```python
from build123d import *

# Parameters (mm, degrees)
SKETCH1_W            = 110
SKETCH1_H            = 60
BOSS_EXTRUDE1_DEPTH  = 10
SKETCH2_W            = 93.6
SKETCH2_H            = 43.6
BOSS_EXTRUDE3_DEPTH  = 7
SKETCH3_W            = 22.1
SKETCH3_H            = 23.4
CUT_EXTRUDE1_DEPTH   = 7
FILLET1_R            = 12
FILLET1_OF_MIRROR1_R = 12
CUT_EXTRUDE3_START   = -10
CUT_EXTRUDE3_DEPTH   = 10


# Read off the part's stored shape, not the designer's step: Cut-Extrude3
with BuildPart() as part:
    # Sketch1 → Boss-Extrude1 (new body)
    with BuildSketch(Plane.XY):
        with Locations((55, 30)):
            Rectangle(SKETCH1_W, SKETCH1_H)
    extrude(amount=BOSS_EXTRUDE1_DEPTH)

    # Sketch2 → Boss-Extrude3 (add)
    with BuildSketch(Plane.XY.offset(10)):
        with Locations((55, 30)):
            Rectangle(SKETCH2_W, SKETCH2_H)
    extrude(amount=BOSS_EXTRUDE3_DEPTH)

    # Sketch3 → Cut-Extrude1 (cut)
    with BuildSketch(Plane.XY.offset(17)):
        with Locations((37.45, 19.9)):
            Rectangle(SKETCH3_W, SKETCH3_H)
    cut_extrude1 = extrude(amount=-CUT_EXTRUDE1_DEPTH, mode=Mode.SUBTRACT)

    # Fillet1
    fillet1_edges = [part.edges().sort_by_distance(p)[0] for p in [
        (26.4, 31.6, 13.5),
    ]]
    fillet(fillet1_edges, radius=FILLET1_R)

    # Mirror1: Cut-Extrude1 across plane
    add(cut_extrude1.mirror(Plane(origin=(55, 0, 0), x_dir=(0, 0, 1), z_dir=(1, 0, 0))), mode=Mode.SUBTRACT)

    # Fillet1 of Mirror1
    fillet1_of_mirror1_edges = [part.edges().sort_by_distance(p)[0] for p in [
        (83.6, 31.6, 13.5),
    ]]
    fillet(fillet1_of_mirror1_edges, radius=FILLET1_OF_MIRROR1_R)

    # Cut-Extrude3 outline → Cut-Extrude3 (cut)
    with BuildSketch(Plane.XY.offset(17).offset(CUT_EXTRUDE3_START)):
        with BuildLine():
            Line((61.3, 31.6), (61.3, 8.4))
            Line((61.3, 8.4), (55, 8.4))
            Line((55, 8.4), (55, 8.2))
            Line((55, 8.2), (61.5, 8.2))
            Line((61.5, 8.2), (61.5, 31.4))
            Line((61.5, 31.4), (71.4, 31.4))
            ThreePointArc((71.4, 31.4), (79.885281374, 27.885281374), (83.4, 19.4))
            Line((83.4, 19.4), (83.4, 8.2))
            Line((83.4, 8.2), (83.6, 8.2))
            Line((83.6, 8.2), (83.6, 19.6))
            ThreePointArc((83.6, 19.6), (80.085281374, 28.085281374), (71.6, 31.6))
            Line((71.6, 31.6), (61.3, 31.6))
        make_face()
    cut_extrude3 = extrude(amount=CUT_EXTRUDE3_DEPTH, mode=Mode.SUBTRACT)

    # Mirror2: Cut-Extrude3 across plane
    add(cut_extrude3.mirror(Plane(origin=(55, 0, 0), x_dir=(0, 0, 1), z_dir=(1, 0, 0))), mode=Mode.SUBTRACT)


solid = part.part
```
Work out the finished part from the listing and answer in its coordinate system (mm). A direction names the side the tool comes from. Give positions to 0.01 mm unless a question says otherwise; leave off trailing zeros. Order: outer loops, then holes, each group sorted by start corner. A loop starts at its lowest first (then second) coordinate and runs counter-clockwise, first axis right, second up.
1. Each of these flat-tipped pins is pushed along its axis until it touches: P1, Ø3, axis at x = 17, y = 50.5, coming from the -Z side; P2, Ø3, axis at x = 56.5, z = 12, coming from the +Y side; P3, Ø3, axis at y = 22, z = 14, coming from the +X side; P4, Ø7.5, axis at y = 30, z = 14.5, coming from the -X side. Where does it stop, or does it pass through?
Result sheet:
P1: stops at z = 0
P2: stops at y = 51.8
P3: stops at x = 101.8
P4: stops at x = 8.2
2. Section A-A, the plane y = 14.5 is taken. Determine the outline of the cut face in (x, z), and give its area (3 significant figures).
Result sheet:
outline: (0, 0) - (110, 0) - (110, 10) - (101.8, 10) - (101.8, 17) - (83.6, 17) - (83.6, 7) - (83.4, 7) - (83.4, 10) - (61.5, 10) - (61.5, 7) - (61.3, 7) - (61.3, 17) - (48.7, 17) - (48.7, 7) - (48.5, 7) - (48.5, 10) - (26.6, 10) - (26.6, 7) - (26.4, 7) - (26.4, 17) - (8.2, 17) - (8.2, 10) - (0, 10) - close
area: 1,440 mm2
3. For faces 4 (the flat face through (54, 30, 0)), 5 (the flat face through (54, 51.8, 13)), 6 (the flat face through (8.2, 30, 13)), 7 (the flat face through (61.5, 20, 8)), determine the directions among +Z, -Z, +X, -X, +Y, -Y from which every point of the face is accessible in a straight line to the end or side of a thin tool.
Result sheet:
face 4: -Z, +X, -X, +Y, -Y
face 5: +Z, +X, -X, +Y
face 6: +Z, -X, +Y, -Y
face 7: +Z
4. Section B-B, the plane z = 12 is taken. Determine the outline of the cut face in (x, y), and give its area (3 significant figures).
Result sheet:
outline: (8.2, 8.2) - (26.4, 8.2) - (26.4, 19.6) arc R12 cw to (38.4, 31.6) - (48.7, 31.6) - (48.7, 8.4) - (61.3, 8.4) - (61.3, 31.6) - (71.6, 31.6) arc R12 cw to (83.6, 19.6) - (83.6, 8.2) - (101.8, 8.2) - (101.8, 51.8) - (8.2, 51.8) - close
area: 3,100 mm2
5. Section C-C, the plane x = 25 is taken. Determine the outline of the cut face in (y, z).
Result sheet:
outline: (0, 0) - (60, 0) - (60, 10) - (51.8, 10) - (51.8, 17) - (8.2, 17) - (8.2, 10) - (0, 10) - close
6. Straight lines are drawn through the part: L1, parallel to X at y = 8.5, z = 14; L2, parallel to Y at x = 40.5, z = 7.75; L3, parallel to X at y = 23, z = 10.5. For each, find the intervals that lie inside material, in ascending order.
Result sheet:
L1: x = 8.2 to 26.4, 48.7 to 61.3, 83.6 to 101.8
L2: y = 0 to 31.4, 31.6 to 60
L3: x = 8.2 to 26.89, 48.7 to 61.3, 83.11 to 101.8
7. The mould has two halves that part along X. Classify faces 1 (the flat face through (54, 35, 17)), 2 (the flat face through (83.4, 14, 8)), 3 (the flat face through (110, 30, 5)): released by +X, released by -X, zero draft, split by the parting line, or undercut.
Result sheet:
face 1: zero draft
face 2: undercut
face 3: released by +X
8. Section D-D, the plane x = 58.5 is taken. Determine the outline of the cut face in (y, z).
Result sheet:
outline: (0, 0) - (60, 0) - (60, 10) - (51.8, 10) - (51.8, 17) - (8.4, 17) - (8.4, 7) - (8.2, 7) - (8.2, 10) - (0, 10) - close
